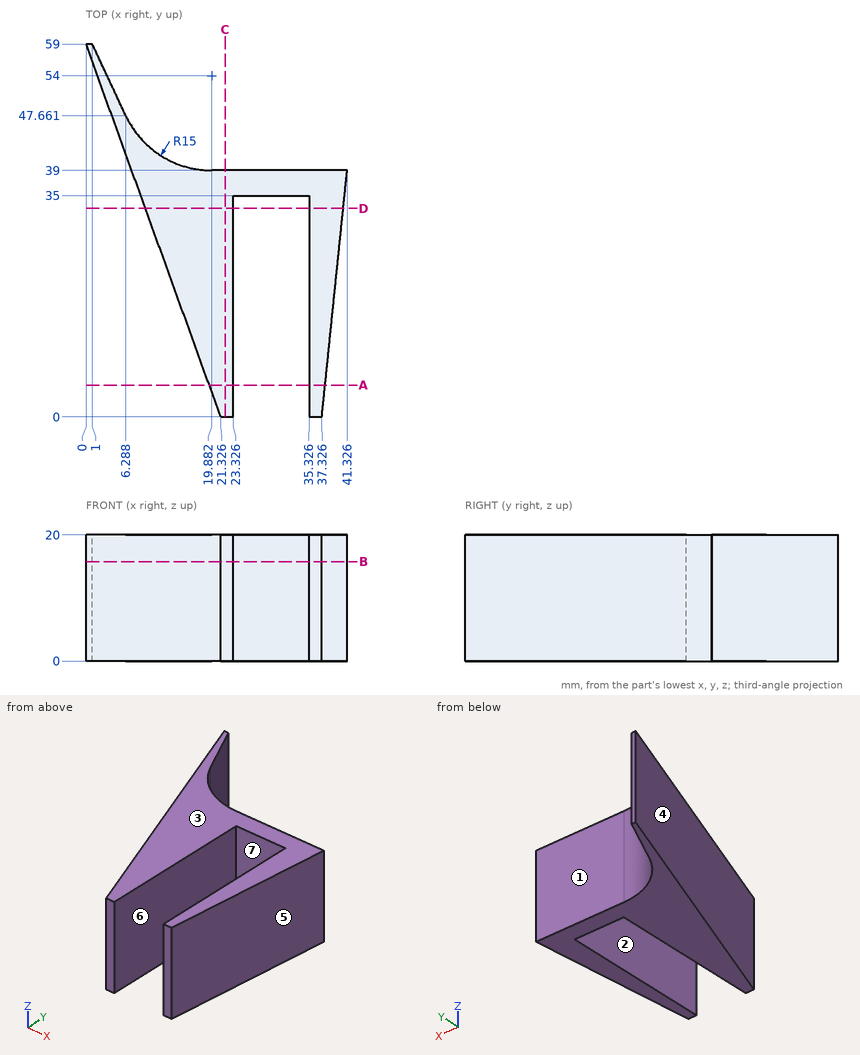
Input: dimensioned drawing with shaded views. Units: mm. Origin: part minimum x, y, z. A direction names the side the tool comes from. Round coordinates to 2 decimals unless told otherwise and drop trailing zeros. Order: outer loops, then holes, each group sorted by start corner. A loop starts at its lowest first (then second) coordinate and runs counter-clockwise, first axis right, second up. Notation, with made-up numbers: (20, 13) -> (61, 13) arc R33 ccw to (61, 48) -> close; hole circle Ø11 at (63.25, 8). An arc over 180 degrees is marked (long way). Put each result on its own line as item: value. Start each with the question number.
Q1. Section B-B on z = 15.75. Return the cut outline in (x, y).
Q2. Section D-D on y = 33. Return the cut outline in (x, z), and give its area (3 significant figures).
Q3. Line query: probe 1 along Y at (x, z) = (22, 18.75); probe 2 along Y at (x, z) = (35, 10.25); probe 3 along X at (y, z) = (34.5, 7) (1 decimal). Output: solid intervals per line, ascending.
Q4. Section C-C on x = 22. Return the cut outline in (y, z), and give its area (3 significant figures).
Q5. Pull-direction query (X, two-part tool) for the marked faces 4, 5, 6 and 7; classes: +X half, -X half, draft (parallel to the pull), parting line (faces both ways), or undercut.
Q6. First-contact query: pin 1 (10 mm diameter, centred on y = 25, z = 7.5, fed in from -X); pin 2 (9.5 mm diameter, centred on x = 26.5, z = 12.5, fed in from -Y); pin 3 (4 mm diameter, centred on y = 8, z = 6.5, fed in from -X); pin 4 (5 mm diameter, centred on x = 27, z = 16.5, fed in from +Y). Flat tips, straight axial feed; report the tip coordinate or a pass-through.
Q7. Reachability of the marked faces 1, 2 and 3 from +Z, -Z, +X, -X, +Y, -Y: full face, straight path, thin tool, end or side. Return the list, or none.
Q8. Section A-A on y = 5. Return the cut outline in (x, z), and give its area (3 significant figures).
Ans:
1. outline: (0, 59) -> (21.33, 0) -> (23.33, 0) -> (23.33, 35) -> (35.33, 35) -> (35.33, 0) -> (37.33, 0) -> (41.33, 39) -> (19.88, 39) arc R15 cw to (6.29, 47.66) -> (1, 59) -> close
2. outline: (9.4, 0) -> (23.33, 0) -> (23.33, 20) -> (9.4, 20) -> close; (35.33, 0) -> (40.71, 0) -> (40.71, 20) -> (35.33, 20) -> close
2. area: 386 mm2
3. probe 1: y = 0 to 39
3. probe 2: y = 35 to 39
3. probe 3: x = 8.9 to 23.3, 35.3 to 40.9
4. outline: (0, 0) -> (39, 0) -> (39, 20) -> (0, 20) -> close
4. area: 780 mm2
5. face 4: -X half
5. face 5: +X half
5. face 6: undercut
5. face 7: undercut
6. pin 1: stops at x = 10.48
6. pin 2: stops at y = 0
6. pin 3: stops at x = 17.71
6. pin 4: stops at y = 39
7. face 1: +Z, -Z, +X, +Y
7. face 2: +Z, -Z, -Y
7. face 3: +Z, +X, -X, +Y, -Y
8. outline: (19.52, 0) -> (23.33, 0) -> (23.33, 20) -> (19.52, 20) -> close; (35.33, 0) -> (37.84, 0) -> (37.84, 20) -> (35.33, 20) -> close
8. area: 126 mm2
